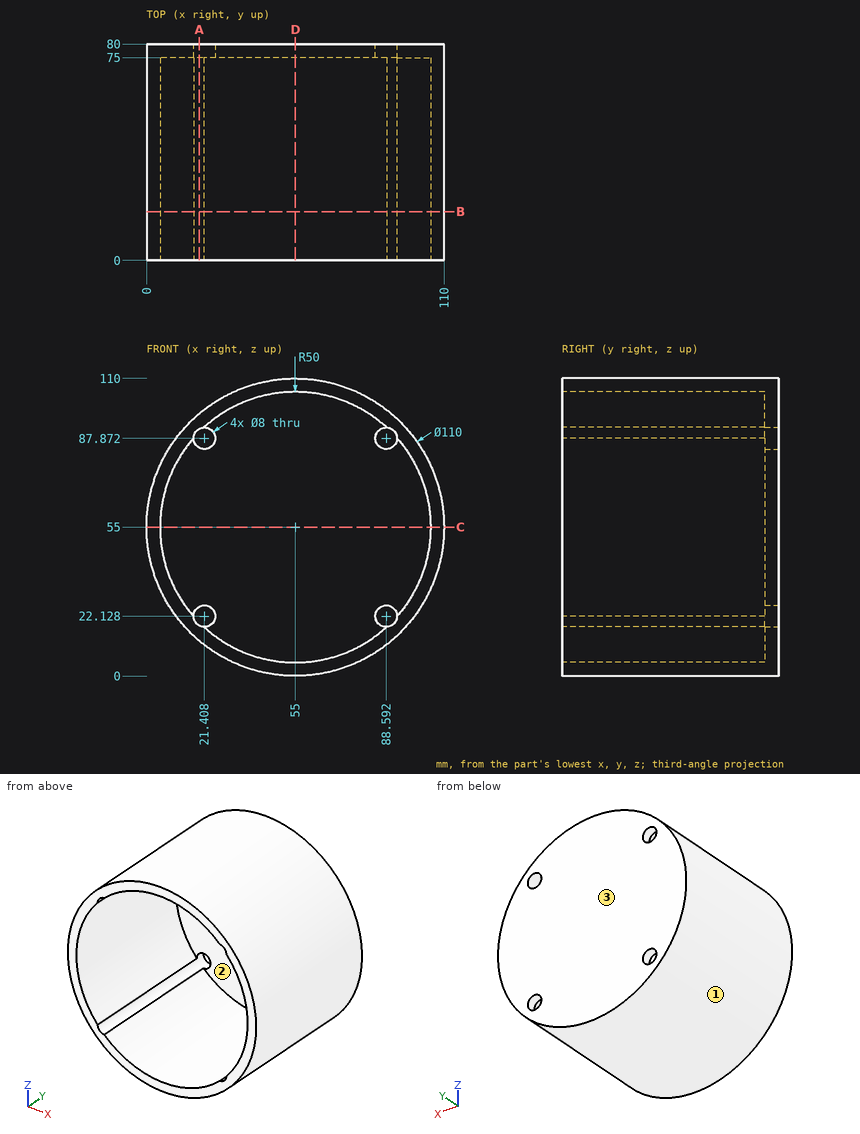
Could you check a few things on this drawing? It's one solid part, dimensions in mm from its lowest x, y, z. Round coordinates to 2 decimals unless told otherwise and drop trailing zeros. Order: outer loops, then holes, each group sorted by start corner. A loop starts at its lowest first (then second) coordinate and runs counter-clockwise, first axis right, second up.
(1) Imagine slicing it at A-A (x = 19.5). Write out the boundary of the cut face in (y, z), plus the area to 3 significant figures.
Response values:
outline: (0, 12.99) - (80, 12.99) - (80, 18.61) - (0, 18.61) - close; (0, 91.39) - (80, 91.39) - (80, 97.01) - (0, 97.01) - close; (75, 25.64) - (80, 25.64) - (80, 84.36) - (75, 84.36) - close
area: 1,190 mm2
(2) I'm going to push flat-ended pins straight in: pin 1 (4 mm diameter, centred on y = 35.5, z = 49.5, fed in from +X); pin 2 (5 mm diameter, centred on x = 64.5, z = 89, fed in from -Y); pin 3 (6 mm diameter, centred on y = 71.5, z = 77.5, fed in from +X); pin 4 (9 mm diameter, centred on x = 21.41, z = 87.87, fed in from +Y). Where does each tip first touch, or does it pass through?
Response values:
pin 1: stops at x = 109.89
pin 2: stops at y = 75
pin 3: stops at x = 106.43
pin 4: stops at y = 80
(3) Imagine slicing it at C-C (z = 55). Write out the boundary of the cut face in (x, y).
Response values:
outline: (0, 0) - (5, 0) - (5, 75) - (105, 75) - (105, 0) - (110, 0) - (110, 80) - (0, 80) - close
(4) Imagine slicing it at D-D (x = 55). Write out the boundary of the cut face in (y, z), plus the area to 3 significant figures.
Response values:
outline: (0, 0) - (80, 0) - (80, 110) - (0, 110) - (0, 105) - (75, 105) - (75, 5) - (0, 5) - close
area: 1,300 mm2
(5) If we mould it in two halves opening along Z, with no side actions, what happens to the marked faces 1, 2 and 3? For each: released by +Z, released by -Z, zero draft, split by the parting line, or undercut.
Response values:
face 1: split by the parting line
face 2: undercut
face 3: zero draft
(6) Imagine slicing it at B-B (y = 18). Write out the boundary of the cut face in (x, z) (1 decimal).
Response values:
outline: circle Ø110 at (55, 55); hole (17.4, 22) arc R4 ccw to (21.2, 18.1) arc R50 ccw to (88.8, 18.1) arc R4 ccw to (92.6, 22) arc R50 ccw to (92.6, 88) arc R4 ccw to (88.8, 91.9) arc R50 ccw to (21.2, 91.9) arc R4 ccw to (17.4, 88) arc R50 ccw to start
(7) Please list where these lines run through material, in increasing order: line 1 along Z through (x, y) = (56, 35); line 2 along Y through (x, z) = (96.5, 43); line 3 along X through (y, z) = (66, 23).
Response values:
line 1: z = 0.01 to 5.01, 104.99 to 109.99
line 2: y = 75 to 80
line 3: x = 10.27 to 16.58, 93.42 to 99.73
